The listing builds one solid part. Answer for the finished solid, in the listing's coordinates (mm). Face numbers are marked on the shaded views. A direction names the side the tool comes from. Give positions to 0.01 mm unless a question says otherwise; leave off trailing zeros. Loops run counter-clockwise (first coordinate to the right, second up) from the corner with the lowest first, then second, coordinate; pieces in that order, holes last. Notation, with made-up numbers: M 78.25,-36 L 103.25,-36 A18 cw 103.25,-5 Z; hole C -35,15 d7. An arc over 180 degrees is marked long. One line per item, written item: value. Start each with the question number.
Q1. For the marked faces 4, 5 and 6, determine the directions among +Z, -Z, +X, -X, +Y, -Y from which every point of the face is accessible in a straight line to the end or side of a thin tool.
Q2. A cutting plane is placed at C-C, the plane x = 0. Determine the outline of the cut face in (y, z) (3 decimals), and give its area (3 significant figures).
Q3. Flat-ended cylindrical pins translate along their axes: pin 1 (5.5 mm diameter, centred on y = -163.5, z = -1.5, fed in from +X); pin 2 (24 mm diameter, centred on x = 3.5, y = -169, fed in from -Z); pin 3 (3 mm diameter, centred on x = -24.5, y = -29.5, fed in from +Z). Find the tip coordinate at first contact, or state that the pin passes through.
Q4. A cutting plane is placed at A-A, the plane z = 0. Determine the outline of the cut face in (x, y) (3 decimals).
Q5. A cutting plane is placed at D-D, the plane y = -71. Determine the outline of the cut face in (x, z).
Q6. A cutting plane is placed at B-B, the plane y = -148. Determine the outline of the cut face in (x, z).
Q7. Consider L1, parallel to Z at x = -0.5, y = -8.5; L2, parallel to Y at x = 21.5, z = -6 (3 decimals); L3, parallel to Z at x = 21, y = -42. Determine where each line is inside the solid, lowest interval first.
Q8. The mould has two halves that part along Z. Classify the marked faces 1, 2 and 3: +Z half, -Z half, draft (parallel to the pull), parting line (faces both ways), or undercut.
from build123d import *

# Parameters (mm, degrees)
BOSS_EXTRUDE2_START = -142.995
BOSS_EXTRUDE2_DEPTH = 142.995
BOSS_EXTRUDE3_DEPTH = 5
CUT_EXTRUDE2_REACH  = 156.714
SKETCH5_W           = 12
SKETCH5_H           = 12
SKETCH6_W           = 30
SKETCH6_H           = 28
SKETCH6_W_2         = 20
SKETCH6_H_2         = 18
BOSS_EXTRUDE4_DEPTH = 53


with BuildPart() as part:
    # Sketch3 → Boss-Extrude2 (new body)
    with BuildSketch(Plane(origin=(0, 0, 0), x_dir=(-1, 0, 0), z_dir=(0, 1, 0)).offset(BOSS_EXTRUDE2_START)):
        with BuildLine():
            ThreePointArc((-7.414110804, 41.102672806), (-36.485572351, 20.327364833), (-38.852451785, -15.325982549))
            ThreePointArc((-38.852451785, -15.325982549), (17.139485086, -38.087226229), (37.237407808, 18.914920316))
            ThreePointArc((37.237407808, 18.914920316), (18.585783578, 37.402772619), (-7.414110804, 41.102672806))
        make_face()
        with BuildLine():
            ThreePointArc((-34.201246039, -13.49123867), (-0.785346896, -36.757611208), (33.593802773, -14.939717757))
            ThreePointArc((33.593802773, -14.939717757), (13.43775935, 34.22229354), (-34.78367135, 11.909448303))
            ThreePointArc((-34.78367135, 11.909448303), (-36.756338657, -0.842804842), (-34.201246039, -13.49123867))
        make_face(mode=Mode.SUBTRACT)
    extrude(amount=BOSS_EXTRUDE2_DEPTH)

    # Sketch4 → Boss-Extrude3 (add)
    with BuildSketch(Plane.XZ.offset(142.99499992)):
        with BuildLine():
            ThreePointArc((0, 36.765999938), (-30.83028068, -20.030789916), (33.593802773, -14.939717757))
            ThreePointArc((33.593802773, -14.939717757), (30.83028068, 20.030789916), (0, 36.765999938))
        make_face()
    extrude(amount=-BOSS_EXTRUDE3_DEPTH)

    # Sketch5 → Cut-Extrude2 (cut, up to next)
    with BuildSketch(Plane.XZ.offset(142.99499992), mode=Mode.PRIVATE) as cut_extrude2_sk1:
        Rectangle(SKETCH5_W, SKETCH5_H)
    cut_extrude2_tool1 = extrude(cut_extrude2_sk1.sketch, amount=-CUT_EXTRUDE2_REACH, mode=Mode.PRIVATE) & part.part
    add(cut_extrude2_tool1.solids().sort_by_distance((0, -142.995, 0))[0], mode=Mode.SUBTRACT)

    # Sketch6 → Boss-Extrude4 (add)
    with BuildSketch(Plane.XZ.offset(142.99499992)):
        Rectangle(SKETCH6_W, SKETCH6_H)
        Rectangle(SKETCH6_W_2, SKETCH6_H_2, mode=Mode.SUBTRACT)
    extrude(amount=BOSS_EXTRUDE4_DEPTH)


solid = part.part
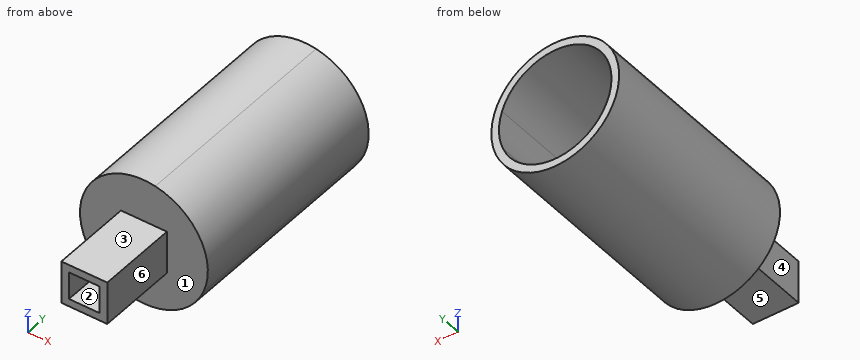
Answer block:
1. face 4: +Z, -Z, -X, -Y
1. face 5: -Z, +X, -X, -Y
1. face 6: +Z, -Z, +X, -Y
2. outline: M -195.995,-14 L -142.995,-14 L -142.995,-41.766 L 0,-41.766 L 0,-36.766 L -137.995,-36.766 L -137.995,-6 L -142.995,-6 L -142.995,-9 L -195.995,-9 Z; M -195.995,9 L -142.995,9 L -142.995,6 L -137.995,6 L -137.995,36.766 L 0,36.766 L 0,41.766 L -142.995,41.766 L -142.995,14 L -195.995,14 Z
2. area: 2,270 mm^2
3. pin 1: x = 15
3. pin 2: z = -14
3. pin 3: z = 34.86
4. outline: M -41.766,-142.995 L -15,-142.995 L -15,-195.995 L -10,-195.995 L -10,-142.995 L -6,-142.995 L -6,-137.995 L -36.766,-137.995 L -36.766,0 L -41.766,0 Z; M 6,-142.995 L 10,-142.995 L 10,-195.995 L 15,-195.995 L 15,-142.995 L 41.766,-142.995 L 41.766,0 L 36.766,0 L 36.766,-137.995 L 6,-137.995 Z
5. outline: C 0,0 d83.53; hole C 0,0 d73.53
6. outline: M -15,-14 L 15,-14 L 15,14 L -15,14 Z; hole M -10,-9 L 10,-9 L 10,9 L -10,9 Z
7. L1: -41.76 to -36.76, 36.76 to 41.76
7. L2: -142.995 to -137.995
7. L3: -36.1 to -30.18, 30.18 to 36.1
8. face 1: draft
8. face 2: undercut
8. face 3: +Z half
